Check sheet for the modelled part. Datum: model origin and axes. Units: mm. A direction names the side the tool comes from. Coordinates: 2 decimals unless noted, no trailing zeros. Order: outer loops, then holes, each group sorted by start corner. A loop starts at its lowest first (then second) coordinate and runs counter-clockwise, first axis right, second up. Notation, with made-up numbers: (61.5, 48) -> (77.5, 48) arc R12 ccw to (77.5, 52) -> close; hole circle Ø3 at (40.5, 60). An arc over 180 degrees is marked (long way). Put each result on its own line as item: value. Start each with the question number.
Autodesk Inventor part; units mm, degrees
ref_plane "YZ Plane" through (0, 0, 0) normal (1, 0, 0) x (0, 1, 0)
ref_plane "XZ Plane" through (0, 0, 0) normal (0, 1, 0) x (-1, 0, 0)
ref_plane "XY Plane" through (0, 0, 0) normal (0, 0, 1) x (1, 0, 0)
sketch "Sketch1" plane through (0, 0, 0) normal (0, 0, 1) x (1, 0, 0)
  line L0 (-750, 0) -> (750, 0) construction
  line L1 (750, 0) -> (750, -2100) construction
  line L2 (750, -2100) -> (110, -2700) construction
  line L3 (108.9077, -2700) -> (-108.9077, -2700) construction
  line L4 (-110, -2700) -> (-750, -2100) construction
  line L5 (-750, -2100) -> (-750, 0) construction
  arc A0 (745.2369, 0.4471) -> (-745.2369, 0.4471) centre (0, -7964.7662) ccw
  arc A1 (-750.6265, -4.7429) -> (-776.2932, -222.5) centre (7180.7944, -1050) ccw
  arc A2 (-777.5832, -235) -> (-778.8534, -247.5) centre (7180.7944, -1050) ccw construction
  arc A3 (750.1285, -2099.0286) -> (778.8534, -247.5) centre (-7180.7944, -1050) ccw construction
  arc A4 (777.5832, -235) -> (776.2932, -222.5) centre (-7180.7944, -1050) ccw
  line L6 (-777.5832, -235) -> (777.5832, -235) construction
  arc A5 (-749.3229, -2100.7083) -> (-677.5699, -2174.8011) centre (5033.2984, 3427.5183) ccw construction
  line L7 (-750, -2100) -> (750, -2100) construction
  line L8 (-547.1729, -2035.7109) -> (-801.0834, -2306.5488) construction
  arc A6 (-677.5699, -2174.8011) -> (-110.8367, -2699.2976) centre (5033.2984, 3427.5183) ccw construction
  arc A7 (-745.2369, 0.4471) -> (-750.6265, -4.7429) centre (-744.6779, -5.5268) ccw
  arc A8 (750.6265, -4.7429) -> (745.2369, 0.4471) centre (744.6779, -5.5268) ccw
  arc A9 (-750.1285, -2099.0286) -> (-749.3229, -2100.7083) centre (-747.1545, -2098.6352) ccw construction
  arc A10 (110.8367, -2699.2976) -> (677.5699, -2174.8011) centre (-5033.2984, 3427.5183) ccw construction
  line L9 (553.8195, -2042.8006) -> (794.4368, -2299.4591) construction
  arc A11 (677.5699, -2174.8011) -> (749.3229, -2100.7083) centre (-5033.2984, 3427.5183) ccw construction
  arc A12 (749.3229, -2100.7083) -> (750.1285, -2099.0286) centre (747.1545, -2098.6352) ccw construction
  arc A13 (-110.8367, -2699.2976) -> (-108.9077, -2700) centre (-108.9077, -2697) ccw construction
  arc A14 (108.9077, -2700) -> (110.8367, -2699.2976) centre (108.9077, -2697) ccw construction
  line L10 (-778.8534, -247.5) -> (778.8534, -247.5) construction
  line L11 (-776.2932, -222.5) -> (776.2932, -222.5) construction
  arc A15 (-776.2932, -222.5) -> (-777.5832, -235) centre (7180.7944, -1050) ccw
  arc A16 (-778.8534, -247.5) -> (-750.1285, -2099.0286) centre (7180.7944, -1050) ccw construction
  arc A17 (778.8534, -247.5) -> (777.5832, -235) centre (-7180.7944, -1050) ccw construction
  arc A18 (776.2932, -222.5) -> (750.6265, -4.7429) centre (-7180.7944, -1050) ccw
  point P0 (0, 0)
  point P1 (0, 0)
  point P2 (0, -2700)
  point P3 (-674.1281, -2171.1299)
  point P4 (674.1281, -2171.1299)
  dimension "d17" = 1500
  dimension "d18" = 2100
  dimension "d19" = 220
  dimension "d20" = 2700
  dimension "d21" = 8000
  dimension "d31" = 8000
  dimension "d33" = 8000
  dimension "d34" = 235
  dimension "d35" = 8000
  dimension "d36" = 104
  dimension "d37" = 6
  dimension "d40" = 3
  dimension "d41" = 8000
  dimension "d42" = 104
  dimension "d44" = 3
  dimension "d46" = 12.5
  dimension "d47" = 12.5
contour flange "Contour Flange1" sketch "Sketch1" thickness 3 bend radius 3 width 1000 along (0, 0, 1) mid plane no both sides no wall seen from (776.9407, -228.7497, 0) lies toward (-0.9947169, -0.1026563, 0) curves A4 A18 A8 A0 A7 A1 A15
bend "Bend1"
corner "Corner1"
equation "\"d17\" = Бак_ширина_общая"
equation "\"d18\" = Бак_высота_до_конуса"
equation "\"d19\" = Бак_брюхо_ширина_полки"
equation "\"d21\" = Бак_радиус_стенок_общий"
equation "\"d31\" = Бак_радиус_стенок_общий"
equation "\"d33\" = Бак_радиус_стенок_общий"
equation "\"d34\" = Бак_спина_длина_фланцев"
equation "\"d35\" = Бак_радиус_стенок_общий"
equation "\"d37\" = Thickness + BendRadius"
equation "\"d40\" = Thickness"
equation "\"d41\" = Бак_радиус_стенок_общий"
equation "\"d46\" = Бак_нахлест_фланца"
equation "\"d47\" = Бак_нахлест_фланца"
equation "\"d3\" = Thickness"
equation "\"d4\" = BendReliefWidth"
equation "\"d5\" = BendReliefDepth"
equation "\"d6\" = MinimumRemnant"
equation "\"d7\" = TransitionRadius"
equation "\"d9\" = BendRadius"
equation "\"d11\" = CornerReliefSize"
equation "\"d12\" = GapSize"
equation "\"d13\" = JacobiRadiusSize"
equation "\"BendRadius\" = Thickness"
equation "\"BendReliefWidth\" = Thickness"
equation "\"BendReliefDepth\" = 0.5 * Thickness"
equation "\"CornerReliefSize\" = 4 * Thickness"
equation "\"MinimumRemnant\" = 2 * Thickness"
equation "\"TransitionRadius\" = BendRadius"
equation "\"JacobiRadiusSize\" = BendRadius"
equation "\"GapSize\" = Thickness"
properties part number "МОО 010 лист спина 1" material "Stainless Steel AISI 304"
1) Sectioned sample at A-A (y = -202). Record the boundary of the cut face in (x, z).
2) Sectioned sample at C-C (y = -38.5). Record the boundary of the cut face in (x, z), plus the area to 3 significant figures.
3) Scan lines: line 1 along X through (y, z) = (-128.5, 272.5); line 2 along X through (y, z) = (-64, 393.5); line 3 along Y through (x, z) = (-503, 915.5). Record each from-to range of solid material in increasing order. Write a range as [from, to].
4) Gauge pin test, flat ends, axial feed: pin 1 (4 mm diameter, centred on y = -156, z = 229.5, fed in from +X); pin 2 (10 mm diameter, centred on y = -50, z = 141.5, fed in from +X); pin 3 (1.5 mm diameter, centred on y = -152, z = 724.5, fed in from +X). Record the tip position at first contact, or that the pin passes through.
5) Sectioned sample at D-D (x = -405). Record the boundary of the cut face in (y, z).
6) Sectioned sample at B-B (z = 812). Record the boundary of the cut face in (x, y).
7) Access from +Z, -Z, +X, -X, +Y, -Y to the whole of each face (thin tool, end or side, straight path). Record for faces 1 (the cylindrical face through (764.026, -112.009, 493)), 2 (the cylindrical face through (-761.406, -115.408, 493)).
Entries:
1. outline: (-774.13, 0) -> (-771.12, 0) -> (-771.12, 1000) -> (-774.13, 1000) -> close; (771.12, 0) -> (774.13, 0) -> (774.13, 1000) -> (771.12, 1000) -> close
2. outline: (-755, 0) -> (-751.98, 0) -> (-751.98, 1000) -> (-755, 1000) -> close; (751.98, 0) -> (755, 0) -> (755, 1000) -> (751.98, 1000) -> close
2. area: 6,050 mm2
3. line 1: x = [-765.96, -762.94], [762.94, 765.96]
3. line 2: x = [-758.21, -755.19], [755.19, 758.21]
3. line 3: y = [16.4, 19.41]
4. pin 1: stops at x = 769.32
4. pin 2: stops at x = 757.09
4. pin 3: stops at x = 768.73
5. outline: (21.97, 0) -> (24.98, 0) -> (24.98, 1000) -> (21.97, 1000) -> close
6. outline: (-777.58, -235) -> (-774.6, -235.31) arc R7966.73 cw to (-773.31, -222.81) arc R7996.81 cw to (-747.65, -5.13) arc R3 cw to (-744.96, -2.54) arc R7997 cw to (744.96, -2.54) arc R3 cw to (747.65, -5.13) arc R7997.19 cw to (773.31, -222.81) arc R8027.5 cw to (774.6, -235.31) -> (777.58, -235) arc R8030.5 ccw to (776.29, -222.5) arc R8000.19 ccw to (750.63, -4.74) arc R6 ccw to (745.24, 0.45) arc R8000 ccw to (-745.24, 0.45) arc R6 ccw to (-750.63, -4.74) arc R7999.81 ccw to (-776.29, -222.5) arc R7969.73 ccw to start
7. face 1: +Z, -Z, +X, +Y
7. face 2: +Z, -Z, -Y
